Work out the finished part from the listing and answer in its coordinate system (mm). A direction names the side the tool comes from. Coordinates: 2 decimals unless noted, no trailing zeros. Order: outer loops, then holes, each group sorted by start corner. A loop starts at its lowest first (then second) coordinate and runs counter-clockwise, first axis right, second up.
1. The part is cut by section B-B, the plane y = -6. Give the vertices of the cut face in (x, z).
2. The part is cut by section C-C, the plane z = 4.25. Give the vertices of the cut face in (x, y).
3. The part is cut by section A-A, the plane z = 0. Give the vertices of the cut face in (x, y), then the cut area to 3 significant figures.
4. The part is cut by section D-D, the plane y = -3.75. Give the vertices of the cut face in (x, z), then the cut area to 3 significant figures.
5. A tool of negligible diameter and unlimited length cuts with its end or side. For faces 1 (the flat face through (0, -2, 0)), 2 (the flat face through (-29, 10, 0)), 3 (the flat face through (-26.5, 6.9, -1.4)), from which of +Z, -Z, +X, -X, +Y, -Y can it reach the whole face along a straight path? Write none if from no direction.
6. Flat-ended cylindrical pins translate along their axes: pin 1 Ø6 at (x, z) = (-5.5, 0) entering from +Y; pin 2 Ø3 at (y, z) = (-4, 3.5) entering from +X; pin 3 Ø6 at (x, z) = (1, 0) entering from -Y. Find the tip coordinate at first contact, or state that the pin passes through.
7. Find the intervals of material crossed by probe 1 along Y at (x, z) = (-30, 0); probe 2 along X at (y, z) = (4.5, 2.5); probe 3 along Y at (x, z) = (2.5, -1.25), in increasing order.
8. Determine the mould class of faces 4 (the cylindrical face through (-28.965, -7.464, -0.325)), 5 (the flat face through (-9, 0, 6)), 6 (the flat face through (-26.5, -5.1, -1.4)), 7 (the flat face through (-9, 0, -6)) for opening direction Z: +Z half, -Z half, draft (parallel to the pull), parting line (faces both ways), or undercut.
```python
from build123d import *

# Parameters (mm, degrees)
SKETCH_1_W      = 53
SKETCH_1_H      = 12
EXTRUDE_1_DEPTH = 2
SKETCH_2_W      = 12
SKETCH_2_H      = 20
SKETCH_2_R      = 1.5
EXTRUDE_2_DEPTH = 5


with BuildPart() as part:
    # 草图1 → 凸台-拉伸1 (new, symmetric)
    with BuildSketch(Plane(origin=(0, 0, 0), x_dir=(1, 0, 0), z_dir=(0, 1, 0))):
        Rectangle(SKETCH_1_W, SKETCH_1_H)
    extrude(amount=EXTRUDE_1_DEPTH, both=True)

    # 草图2 → 凸台-拉伸2 (add)
    with BuildSketch(Plane.ZY.offset(26.5)):
        Rectangle(SKETCH_2_W, SKETCH_2_H)
        with Locations((0, 6)):
            Circle(SKETCH_2_R, mode=Mode.SUBTRACT)
        with Locations((0, -6)):
            Circle(SKETCH_2_R, mode=Mode.SUBTRACT)
    extrude(amount=EXTRUDE_2_DEPTH)


solid = part.part
```
Geometry says:
1. outline: (-31.5, -6) - (-26.5, -6) - (-26.5, -1.5) - (-31.5, -1.5) - close; (-31.5, 1.5) - (-26.5, 1.5) - (-26.5, 6) - (-31.5, 6) - close
2. outline: (-31.5, -10) - (-26.5, -10) - (-26.5, -2) - (26.5, -2) - (26.5, 2) - (-26.5, 2) - (-26.5, 10) - (-31.5, 10) - close
3. outline: (-31.5, -10) - (-26.5, -10) - (-26.5, -7.5) - (-31.5, -7.5) - close; (-31.5, -4.5) - (-26.5, -4.5) - (-26.5, -2) - (26.5, -2) - (26.5, 2) - (-26.5, 2) - (-26.5, 4.5) - (-31.5, 4.5) - close; (-31.5, 7.5) - (-26.5, 7.5) - (-26.5, 10) - (-31.5, 10) - close
3. area: 282 mm2
4. outline: (-31.5, -6) - (-26.5, -6) - (-26.5, 6) - (-31.5, 6) - close
4. area: 60.0 mm2
5. face 1: +Z, -Z, +X, -Y
5. face 2: +Z, -Z, +X, -X, +Y
5. face 3: +Z, -Z, +X, +Y
6. pin 1: stops at y = 2
6. pin 2: stops at x = -26.5
6. pin 3: stops at y = -2
7. probe 1: y = -10 to -7.5, -4.5 to 4.5, 7.5 to 10
7. probe 2: x = -31.5 to -26.5
7. probe 3: y = -2 to 2
8. face 4: undercut
8. face 5: +Z half
8. face 6: draft
8. face 7: -Z half
